```python
from build123d import *

# Parameters (mm, degrees)
SKETCH_1_W          = 90
SKETCH_1_H          = 70
EXTRUDE_1_DEPTH     = 10
FILLET_1_R          = 10
SKETCH_2_R          = 8.935644791
CUT_EXTRUDE_1_DEPTH = 10


with BuildPart() as part:
    # 草图1 → 凸台-拉伸1 (new body)
    with BuildSketch(Plane(origin=(0, 0, 0), x_dir=(1, 0, 0), z_dir=(0, 1, 0))):
        Rectangle(SKETCH_1_W, SKETCH_1_H)
    extrude(amount=EXTRUDE_1_DEPTH)

    # 圆角1
    fillet_1_edges = [part.edges().sort_by_distance(p)[0] for p in [
        (45, 5, 35),
        (-45, 5, 35),
        (-45, 5, -35),
        (45, 5, -35),
    ]]
    fillet(fillet_1_edges, radius=FILLET_1_R)

    # 草图2 → 切除-拉伸1 (cut)
    with BuildSketch(Plane(origin=(0, 10, 0), x_dir=(1, 0, 0), z_dir=(0, 1, 0))):
        with Locations(Location((0, 19.345170793, 0), (0, 0, 270))):
            Circle(SKETCH_2_R)
        with Locations(Location((0, -19.345170793, 0), (0, 0, 90))):
            Circle(SKETCH_2_R)
    extrude(amount=-CUT_EXTRUDE_1_DEPTH, mode=Mode.SUBTRACT)

    # 草图5 → 旋转1 (revolve)
    with BuildSketch(Plane.XY, mode=Mode.PRIVATE) as revolve_1_sk:
        with BuildLine():
            Line((45, 25), (45, -15))
            ThreePointArc((45, -15), (65, 5), (45, 25))
        make_face()
    revolve(revolve_1_sk.sketch.rotate(Axis((0, 30.833762992, 0), (0, -1, 0)), 90), axis=Axis((0, 30.833762992, 0), (0, -1, 0)))


solid = part.part
```
Read the model definition and answer for the solid it produces. Units are mm, in the model's axes. A direction names the side the tool comes from. Coordinates: 2 decimals unless noted, no trailing zeros. Write each loop counter-clockwise with the first axis right and the second up, starting at its lowest first coordinate (ties: lowest second). Pieces come first, ordered by that corner, then holes. Notation, with made-up numbers: (-22, 55) -> (8, 55) arc R22 cw to (8, 64) -> close; hole circle Ø3 at (13.25, -4). An arc over 180 degrees is marked (long way). Answer as a JSON object with one key per item and string values.
Q1. The part is cut by section B-B on z = 0. Give the vertices of the cut face in (x, y).
The answers:
{"outline": "(-45, -15) -> (-45, 0) -> (45, 0) -> (45, -15) arc R20 ccw to (45, 25) -> (45, 10) -> (-45, 10) -> (-45, 25) arc R20 ccw to start"}
Q2. The part is cut by section C-C on y = 2.5. Give the vertices of the cut face in (x, z), then the cut area to 3 significant figures.
The answers:
{"outline": "circle Ø129.69 at (0, 0); hole (-28.28, -35) arc R45 ccw to (28.28, -35) -> close; hole (-28.28, 35) -> (28.28, 35) arc R45 ccw to start; hole circle Ø17.87 at (0, -19.35); hole circle Ø17.87 at (0, 19.35)", "area": "11,900 mm2"}
Q3. The part is cut by section A-A on x = 0. Give the vertices of the cut face in (y, z).
The answers:
{"outline": "(-15, -45) arc R20 ccw to (25, -45) -> close; (-15, 45) -> (25, 45) arc R20 ccw to start; (0, -35) -> (10, -35) -> (10, -28.28) -> (0, -28.28) -> close; (0, -10.41) -> (10, -10.41) -> (10, 10.41) -> (0, 10.41) -> close; (0, 28.28) -> (10, 28.28) -> (10, 35) -> (0, 35) -> close"}
Q4. Flat-ended cylindrical pins translate along their axes: pin 1 Ø3 at (y, z) = (-9.5, 1) entering from -X; pin 2 Ø11 at (x, y) = (-8.5, 6.5) entering from +Z; pin 3 Ø8 at (y, z) = (-1, 12) entering from -X. Find the tip coordinate at first contact, or state that the pin passes through.
The answers:
{"pin 1": "stops at x = -60.19", "pin 2": "stops at z = 64.92", "pin 3": "stops at x = -64.1"}
Q5. Consider line 1 (Y direction, x = 13, z = -33); line 2 (X direction, y = 13, z = -28.5); line 3 (Z direction, x = 32, y = 14). Determine where each line is inside the solid, lowest interval first. Write a range as [from, to].
The answers:
{"line 1": "y = [0, 10]", "line 2": "x = [-56.56, -34.82], [34.82, 56.56]", "line 3": "z = [-54.11, -31.64], [31.64, 54.11]"}
Q6. The part is cut by section D-D on y = -11. Give the vertices of the cut face in (x, z), then the cut area to 3 significant figures.
The answers:
{"outline": "circle Ø114 at (0, 0); hole circle Ø90 at (0, 0)", "area": "3,850 mm2"}
Q7. A tool of negligible diameter and unlimited length cuts with its end or side. For faces 1 (the cylindrical face through (17.235, 4.72, 41.569)), 2 (the flat face through (-1, 0, 0)), 3 (the flat face through (0, 5, 35)), from which of +Z, -Z, +X, -X, +Y, -Y can it reach the whole face along a straight path? Write none if from no direction.
The answers:
{"face 1": "none", "face 2": "-Y", "face 3": "+Y, -Y"}
Q8. Determine the mould class of faces 4 (the flat face through (0, 5, -35)), 5 (the flat face through (-1, 10, 0)) for opening direction Z: pulls with the +Z half, pulls with the -Z half, needs draft (parallel to the pull), parting line crosses it, or undercut.
The answers:
{"face 4": "undercut", "face 5": "undercut"}
